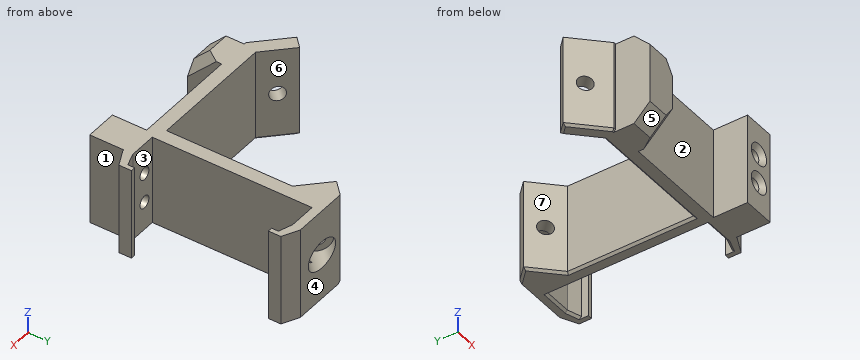
from build123d import *

# Parameters (mm, degrees)
CYLINDER003_R            = 3
CYLINDER003_DEPTH        = 10
PAD008_DEPTH             = 10
SKETCH032_R              = 1.625
POCKET023_DEPTH          = 55.910244
SKETCH033_W              = 20
SKETCH033_H              = 7
PAD009_DEPTH             = 7.5
SKETCH034_R              = 1.375
POCKET024_DEPTH          = 12
CHAMFER020_1_SIZE        = 3.5
CHAMFER020_2_SIZE        = 1
CHAMFER021_SIZE          = 0.5
CHAMFER022_SIZE          = 2
CLONE006_PITCH_ANGLE     = 90
CLONE006_PLACEMENT_ANGLE = 45.000049


with BuildPart() as boardbracketscrewheadcylinder:
    # Cylinder003 → Cylinder003 (new body)
    with BuildSketch(Plane(origin=(0, 0.5, 24), x_dir=(1, 0, 0), z_dir=(0, 0, 1))):
        Circle(CYLINDER003_R)
    extrude(amount=CYLINDER003_DEPTH)


with BuildPart() as clone006:
    # Sketch031 → Pad008 (new body, symmetric)
    with BuildSketch(Plane.YZ):
        Polygon((4.5, 21), (4.5, 24.911688), (-4.23971, 33.651398), (-7.975533, 34.909244), (-9.918525, 32.966252), (-9.211418, 32.259145), (-8.150758, 33.319805), (-5.32233, 31.905592), (-1.07969, 27.662951), (-25.828427, 2.914214), (-30.071068, 7.156854), (-31.485281, 9.985281), (-30.424621, 11.045942), (-31.131728, 11.753048), (-33.07472, 9.810056), (-31.714777, 5.972136), (-4.742641, -21), (4.5, -21), (4.5, -18), (-3.5, -18), (-23, 1.5), (-3.5, 21), align=None)
    extrude(amount=PAD008_DEPTH, both=True)

    # Sketch032 → Pocket023 (cut, through all)
    with BuildSketch(Plane.YX.offset(21)):
        with Locations((0.5, 0)):
            Circle(SKETCH032_R)
    extrude(amount=-POCKET023_DEPTH, mode=Mode.SUBTRACT)

    # Cut001: cut BoardBracketScrewHeadCylinder
    add(boardbracketscrewheadcylinder.part, mode=Mode.SUBTRACT)

    # Sketch033 → Pad009 (new body)
    with BuildSketch(Plane(origin=(0, -12.87132, -12.87132), x_dir=(1, 0, 0), z_dir=(0, -0.707107, -0.707107))):
        with Locations((0, 22.75)):
            Rectangle(SKETCH033_W, SKETCH033_H)
        with Locations((0, -7.5)):
            Rectangle(SKETCH033_W, SKETCH033_H)
    extrude(amount=PAD009_DEPTH)

    # Sketch034 → Pocket024 (cut)
    with BuildSketch(Plane(origin=(0, -18.174621, -18.174621), x_dir=(1, 0, 0), z_dir=(0, -0.707107, -0.707107))):
        with Locations((3.25, 22.75)):
            Circle(SKETCH034_R)
    pocket024 = extrude(amount=-POCKET024_DEPTH, mode=Mode.SUBTRACT)

    # Mirrored002: Pocket024 across Sketch034 V_Axis
    add(pocket024.mirror(Plane(origin=(0, -18.174621, -18.174621), x_dir=(0, -0.707107, -0.707107), z_dir=(1, 0, 0))), mode=Mode.SUBTRACT)

    # Chamfer020 1
    chamfer020_1_edges = [clone006.edges().sort_by_distance(p)[0] for p in [
        (-10, -12.87132, -23.477922),
        (10, -12.87132, -23.477922),
    ]]
    chamfer(chamfer020_1_edges, length=CHAMFER020_1_SIZE)

    # Chamfer020 2
    chamfer020_2_edges = [clone006.edges().sort_by_distance(p)[0] for p in [
        (-1.875, -34.2613, -2.087942),
        (1.875, -34.2613, -2.087942),
    ]]
    chamfer(chamfer020_2_edges, length=CHAMFER020_2_SIZE)

    # Chamfer021
    chamfer021_edges = [clone006.edges().sort_by_distance(p)[0] for p in [
        (10, -4.917893, -20.824747),
        (10, -0.12132, -21),
        (10, 4.5, -19.5),
        (10, 0.5, -18),
        (10, -13.25, -8.25),
        (10, -13.25, 11.25),
        (10, 0.5, 21),
        (10, 4.5, 22.955844),
        (10, -30.778175, 8.571068),
        (10, -27.949747, 5.035534),
        (10, -13.454058, 15.288582),
        (10, -3.20101, 29.784271),
        (10, -6.736544, 32.612698),
    ]]
    chamfer(chamfer021_edges, length=CHAMFER021_SIZE)

    # Chamfer022
    chamfer022_edges = [clone006.edges().sort_by_distance(p)[0] for p in [
        (8.25, -14.108757, -19.765611),
        (-8.25, -14.108757, -19.765611),
    ]]
    chamfer(chamfer022_edges, length=CHAMFER022_SIZE)


with BuildPart() as clone006_1:
    # Clone006 pitch: moved
    add(clone006.part.rotate(Axis((0, 0, 0), (0, 1, 0)), CLONE006_PITCH_ANGLE))


with BuildPart() as clone006_2:
    # Clone006 placement: moved
    add(clone006_1.part.moved(Location((-178, 2, -28))).rotate(Axis((-178, 2, -28), (0, 0, 1)), CLONE006_PLACEMENT_ANGLE))


solid = clone006_2.part
The listing builds one solid part. Answer for the finished solid, in the listing's coordinates (mm). Face numbers are marked on the shaded views. A direction names the side the tool comes from. Coordinates: 2 decimals unless noted, no trailing zeros. Loops run counter-clockwise (first coordinate to the right, second up) from the corner with the lowest first, then second, coordinate; pieces in that order, holes last. Notation, with made-up numbers: (37, -25) -> (54, -25) arc R17 cw to (54, -14) -> close; hole circle Ø2 at (86.25, 88.5). An arc over 180 degrees is marked (long way). Answer in a Markdown table with one row per item. Add a question column.
1. Flat-ended cylindrical pins translate along their axes: P1, Ø4, axis at y = -7.5, z = -26.5, coming from the -X side; P2, Ø1.6, axis at y = 20, z = -24.5, coming from the -X side; P3, Ø1, axis at x = -167.5, z = -28, coming from the +Y side; P4, Ø6, axis at x = -179.5, z = -33, coming from the -Y side. Find the tip coordinate at first contact, or state that the pin passes through.
2. For the marked faces 1, 2, 3 and 4, determine the directions among +Z, -Z, +X, -X, +Y, -Y from which every point of the face is accessible in a straight line to the end or side of a thin tool.
3. The part is cut by section C-C, the plane y = 5. Write down the section's boundary in (x, z).
4. The part is cut by section B-B, the plane x = -179.5. Write down the section's boundary in (y, z), then the cut area to 3 significant figures.
5. Determine the mould class of the marked faces 5, 6 and 7 for opening direction Y: +Y half, -Y half, draft (parallel to the pull), parting line (faces both ways), or undercut.
6. Consider line 1 (X direction, y = -19, z = -31.25); line 2 (X direction, y = -12, z = -23.75); line 3 (X direction, y = -20, z = -27.5). Determine where each line is inside the solid, lowest interval first. Write a range as [from, to].
Answer below:
| question | item | result |
|---|---|---|
| 1 | P1 | x = -195.86 |
| 1 | P2 | x = -166.33 |
| 1 | P3 | y = -13.2 |
| 1 | P4 | y = -23.7 |
| 2 | face 1 | +Z, -Z, +X, -Y |
| 2 | face 2 | +Z, -Z, -Y |
| 2 | face 3 | +Z, -Z |
| 2 | face 4 | +Z, -Z, +X, -X, +Y |
| 3 | outline | (-160.68, -37.5) -> (-160.18, -38) -> (-158.18, -38) -> (-157.68, -37.5) -> (-157.68, -18) -> (-160.68, -18) -> close |
| 4 | outline | (-16.2, -38) -> (-13.7, -38) -> (-13.2, -37.5) -> (-13.2, -18) -> (-16.2, -18) -> close |
| 4 | area | 59.9 mm2 |
| 5 | face 5 | -Y half |
| 5 | face 6 | +Y half |
| 5 | face 7 | undercut |
| 6 | line 1 | [-189, -182], [-158.75, -156.62], [-153.87, -151.75] |
| 6 | line 2 | [-193.7, -189.46], [-160.68, -157.68], [-148.68, -147.68] |
| 6 | line 3 | [-189, -182], [-158.75, -151.75] |
